Part model, mm, in its own coordinate system. Face numbers are marked on the shaded views. Give positions to 0.01 mm unless a question says otherwise; leave off trailing zeros. Order: outer loops, then holes, each group sorted by start corner. A loop starts at its lowest first (then second) coordinate and runs counter-clockwise, first axis right, second up. Notation, with made-up numbers: (-9.75, 21.25) - (37.25, 21.25) arc R16 cw to (37.25, 47.25) - close; hole circle Ø7 at (-14, 86.25). An arc over 180 degrees is marked (long way). One line per item, written item: value.
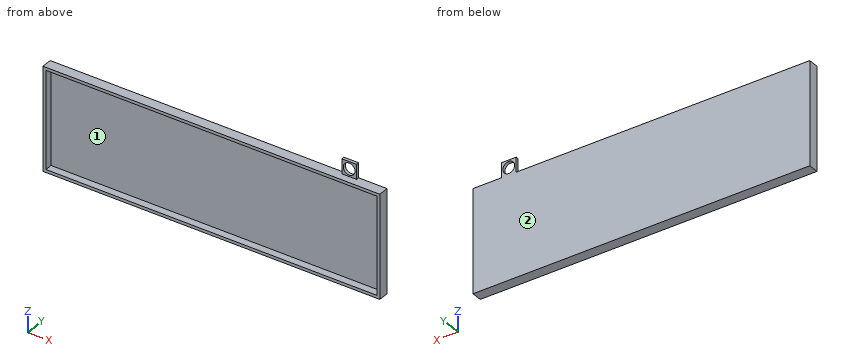
```python
from build123d import *

# Parameters (mm, degrees)
BOSS_EXTRU_1_DEPTH = 70
ESQUISSE3_W        = 224
ESQUISSE3_H        = 5
BOSS_EXTRU_2_DEPTH = 2
ESQUISSE5_W        = 10
ESQUISSE5_H        = 10
ESQUISSE5_R        = 4
BOSS_EXTRU_3_DEPTH = 2
ESQUISSE6_W        = 224
ESQUISSE6_H        = 5
BOSS_EXTRU_4_DEPTH = 2


with BuildPart() as part:
    # Esquisse1 → Boss.-Extru.1 (new body)
    with BuildSketch(Plane.XY):
        Polygon((-115.072635135, 3.126470588), (-115.072635135, -3.873529412), (-113.072635135, -3.873529412), (-113.072635135, 1.126470588), (110.927364865, 1.126470588), (110.927364865, -3.873529412), (112.927364865, -3.873529412), (112.927364865, 3.126470588), align=None)
    extrude(amount=BOSS_EXTRU_1_DEPTH)

    # Esquisse3 → Boss.-Extru.2 (add)
    with BuildSketch(Plane(origin=(0, 0, 0), x_dir=(-1, 0, 0), z_dir=(0, 0, -1))):
        with Locations((1.072635135, -1.373529412)):
            Rectangle(ESQUISSE3_W, ESQUISSE3_H)
    extrude(amount=-BOSS_EXTRU_2_DEPTH)

    # Esquisse5 → Boss.-Extru.3 (add, through all)
    with BuildSketch(Plane.XZ.offset(-1.126470588)):
        with Locations((88.718220762, 75)):
            Rectangle(ESQUISSE5_W, ESQUISSE5_H)
        with Locations(Location((88.718220762, 75, 0), (0, 0, 270))):
            Circle(ESQUISSE5_R, mode=Mode.SUBTRACT)
    extrude(amount=-BOSS_EXTRU_3_DEPTH)

    # Esquisse6 → Boss.-Extru.4 (add)
    with BuildSketch(Plane.XY.offset(70)):
        with Locations((-1.072635135, -1.373529412)):
            Rectangle(ESQUISSE6_W, ESQUISSE6_H)
    extrude(amount=-BOSS_EXTRU_4_DEPTH)


solid = part.part
```
1) Two-plate mould, pull along X, no slides. Class the marked faces 1 and 2: pulls with the +X half, pulls with the -X half, needs draft (parallel to the pull), parting line crosses it, or undercut.
Answer:
face 1: undercut
face 2: needs draft
2) Slice it at B-B on y = -2. Write the cut outline in (x, z).
Answer:
outline: (-115.07, 0) - (112.93, 0) - (112.93, 70) - (-115.07, 70) - close; hole (-113.07, 2) - (110.93, 2) - (110.93, 68) - (-113.07, 68) - close
3) Wall check: line 1 along X through (y, z) = (2.65, 75); line 2 along X through (y, z) = (-3, 24.5); line 3 along Z through (x, y) = (-32, -1.75). Give the ranges that are in metal, low to high. Write a range as [from, to].
Answer:
line 1: x = [83.72, 84.72], [92.72, 93.72]
line 2: x = [-115.07, -113.07], [110.93, 112.93]
line 3: z = [0, 2], [68, 70]
4) Slice it at A-A on z = 75. Write the cut outline in (x, y).
Answer:
outline: (83.72, 1.13) - (84.72, 1.13) - (84.72, 3.13) - (83.72, 3.13) - close; (92.72, 1.13) - (93.72, 1.13) - (93.72, 3.13) - (92.72, 3.13) - close
5) Slice it at C-C on x = -70. Write the cut outline in (y, z), then the cut area to 3 significant figures.
Answer:
outline: (-3.87, 0) - (3.13, 0) - (3.13, 70) - (-3.87, 70) - (-3.87, 68) - (1.13, 68) - (1.13, 2) - (-3.87, 2) - close
area: 160 mm2
6) Drop flat-ended pins along their axis: P1, Ø2, axis at x = -57, y = -1.5, coming from the +Z side; P2, Ø1, axis at y = 2.5, z = 77, coming from the -X side; P3, Ø1, axis at y = 2.5, z = 77.5, coming from the +X side. Give the stop position or say it passes through.
Answer:
P1: stops at z = 70
P2: stops at x = 83.72
P3: stops at x = 93.72
7) Slice it at D-D on z = 51. Write the cut outline in (x, y), then the cut area to 3 significant figures.
Answer:
outline: (-115.07, -3.87) - (-113.07, -3.87) - (-113.07, 1.13) - (110.93, 1.13) - (110.93, -3.87) - (112.93, -3.87) - (112.93, 3.13) - (-115.07, 3.13) - close
area: 476 mm2
